Here's the drawing with two shaded views (mm, measured from the low corner). I have some questions. A direction names the side the tool comes from. Round coordinates to 2 decimals unless told otherwise and drop trailing zeros. Order: outer loops, then holes, each group sorted by start corner. A loop starts at its lowest first (then second) coordinate and runs counter-clockwise, first axis right, second up.
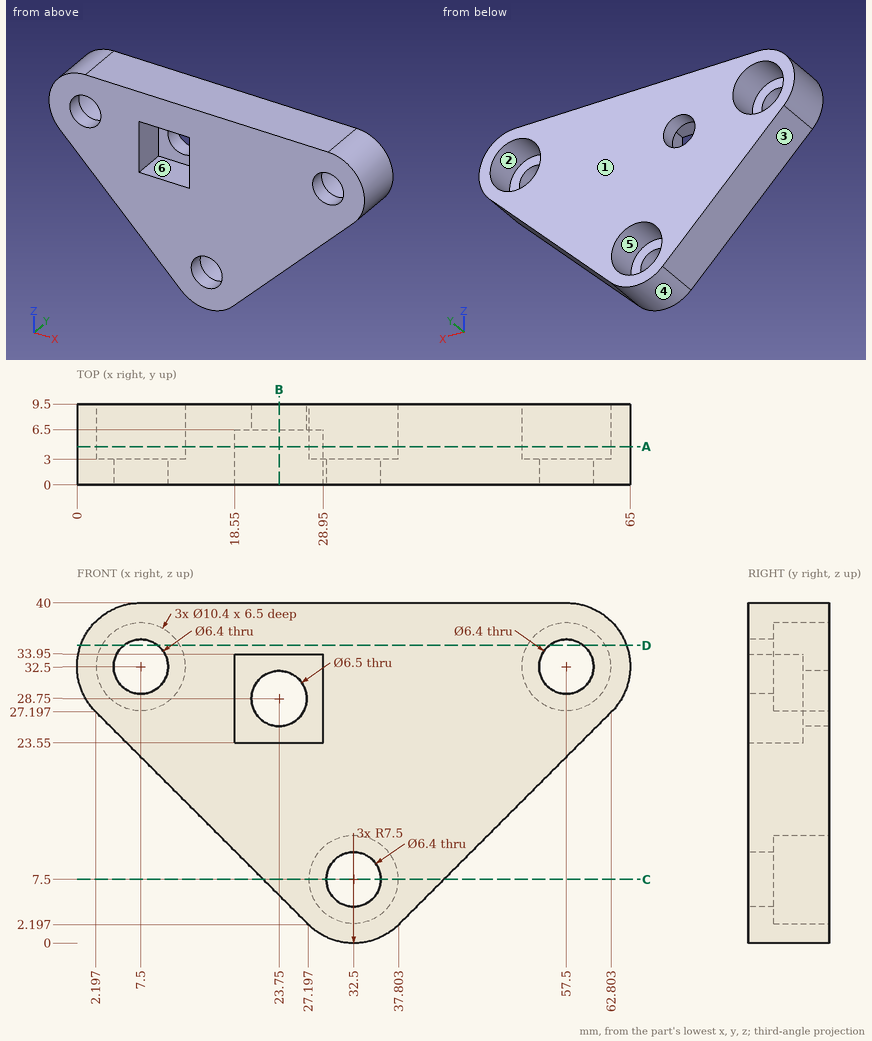
1. If we section it at D-D, the plane z = 35: Write out the boundary of the cut face in (x, y), and give its area (3 significant figures).
Evaluation:
outline: (0.43, 0) - (5.5, 0) - (5.5, 3) - (2.94, 3) - (2.94, 9.5) - (0.43, 9.5) - close; (9.5, 0) - (55.5, 0) - (55.5, 3) - (52.94, 3) - (52.94, 9.5) - (12.06, 9.5) - (12.06, 3) - (9.5, 3) - close; (59.5, 0) - (64.57, 0) - (64.57, 9.5) - (62.06, 9.5) - (62.06, 3) - (59.5, 3) - close
area: 467 mm2
2. If we mould it in two halves opening along X, with no side actions, what happens to the marked faces 1, 2 and 3? For each: released by +X, released by -X, zero draft, split by the parting line, or undercut.
Evaluation:
face 1: zero draft
face 2: undercut
face 3: released by -X
3. If we section it at B-B, the plane x = 23.75: Write out the boundary of the cut face in (y, z).
Evaluation:
outline: (0, 5.64) - (9.5, 5.64) - (9.5, 25.5) - (6.5, 25.5) - (6.5, 23.55) - (0, 23.55) - close; (0, 33.95) - (6.5, 33.95) - (6.5, 32) - (9.5, 32) - (9.5, 40) - (0, 40) - close
4. I'm going to push flat-ended pins straight in: P1, Ø4, axis at y = 7.5, z = 5, coming from the +X side; P2, Ø3, axis at x = 11, y = 4, coming from the -Z side; P3, Ø5, axis at y = 3.5, z = 30.5, coming from the -X side; P4, Ø6, axis at x = 32.5, z = 7.5, coming from the -Y side. Where does each tip first touch, or does it pass through?
Evaluation:
P1: stops at x = 42.61
P2: stops at z = 16.89
P3: stops at x = 0
P4: passes through
5. I need wall thicknesses on probe 1 along X at (y, z) = (1.45, 32.5); probe 2 along Z at (x, y) = (32.5, 2.35); probe 3 along X at (y, z) = (8, 28.75) (1 decimal). Which ranges of each line are inside material? Lowest first, please.
Evaluation:
probe 1: x = 0 to 4.3, 10.7 to 18.55, 28.95 to 54.3, 60.7 to 65
probe 2: z = 0 to 4.3, 10.7 to 40
probe 3: x = 1 to 3.9, 11.1 to 20.5, 27 to 53.9, 61.1 to 64
6. On a 3-axis mill with a long thin cutter (end or side, diameter ignored), from which of +Z, -Z, +X, -X, +Y, -Y can I reach the whole of each face in a straight line? I mean the marked faces 4, 5 and 6. Say none if no direction works.
Evaluation:
face 4: -Z, +Y, -Y
face 5: +Y
face 6: -Y
7. If we section it at C-C, the plane z = 7.5: Write out the boundary of the cut face in (x, y).
Evaluation:
outline: (21.89, 0) - (29.3, 0) - (29.3, 3) - (27.3, 3) - (27.3, 9.5) - (21.89, 9.5) - close; (35.7, 0) - (43.11, 0) - (43.11, 9.5) - (37.7, 9.5) - (37.7, 3) - (35.7, 3) - close
8. If we section it at A-A, the plane y = 4.5: Write out the boundary of the cut face in (x, z), and give its area (3 significant figures).
Evaluation:
outline: (2.2, 27.2) - (27.2, 2.2) arc R7.5 ccw to (37.8, 2.2) - (62.8, 27.2) arc R7.5 ccw to (57.5, 40) - (7.5, 40) arc R7.5 ccw to start; hole circle Ø10.4 at (7.5, 32.5); hole (18.55, 23.55) - (28.95, 23.55) - (28.95, 33.95) - (18.55, 33.95) - close; hole circle Ø10.4 at (32.5, 7.5); hole circle Ø10.4 at (57.5, 32.5)
area: 1,340 mm2
